Can you work these out from the model? Positions are in its coordinate system, mm. A direction names the side the tool comes from. Coordinates: 2 decimals unless noted, no trailing zeros. Loops run counter-clockwise (first coordinate to the right, second up) from the corner with the lowest first, then second, coordinate; pieces in that order, holes last. Notation, with made-up numbers: (-19.5, 7) - (-4.5, 7) arc R22 cw to (-4.5, 36) - close; hole circle Ø9 at (32, 66.25). An arc over 180 degrees is marked (long way). Put each result on its own line as item: value. Start each with the question number.
from build123d import *

# Parameters (mm, degrees)
SKETCH_1_W                  = 230
SKETCH_1_H                  = 150
EXTRUDE_1_DEPTH             = 20
SKETCH_2_W                  = 110
SKETCH_2_H                  = 20
EXTRUDE_2_DEPTH             = 135
FILLET_1_R                  = 55
SKETCH_4_R                  = 27.5
CUT_EXTRUDE_1_DEPTH         = 233.701525564
SKETCH_5_R                  = 11
CUT_EXTRUDE_2_DEPTH         = 193.54869514
PATTERN_LINEAR_1_COUNT      = 2
PATTERN_LINEAR_1_PITCH      = 180
PATTERN_LINEAR_1_COUNT_DIR2 = 2
PATTERN_LINEAR_1_PITCH_DIR2 = 100


with BuildPart() as part:
    # 草图1 → 凸台-拉伸1 (new body)
    with BuildSketch(Plane(origin=(0, 0, 0), x_dir=(1, 0, 0), z_dir=(0, 1, 0))):
        Rectangle(SKETCH_1_W, SKETCH_1_H)
    extrude(amount=EXTRUDE_1_DEPTH)

    # 草图2 → 凸台-拉伸2 (add)
    with BuildSketch(Plane(origin=(0, 20, 0), x_dir=(1, 0, 0), z_dir=(0, 1, 0))):
        with Locations((0, 45)):
            Rectangle(SKETCH_2_W, SKETCH_2_H)
    extrude_2 = extrude(amount=EXTRUDE_2_DEPTH)

    # 镜向1: 凸台-拉伸2 across plane
    add(extrude_2.mirror(Plane.XY))

    # 圆角1
    fillet_1_edges = [part.edges().sort_by_distance(p)[0] for p in [
        (-55, 155, -45),
        (55, 155, -45),
        (-55, 155, 45),
        (55, 155, 45),
    ]]
    fillet(fillet_1_edges, radius=FILLET_1_R - 0.0001)  # a hair under: the kernel refuses the full size

    # 草图4 → 切除-拉伸1 (cut, through all)
    with BuildSketch(Plane.XY.offset(55)):
        with Locations((0, 100)):
            Circle(SKETCH_4_R)
    extrude(amount=-CUT_EXTRUDE_1_DEPTH, mode=Mode.SUBTRACT)

    # 草图5 → 切除-拉伸2 (cut, through all)
    with BuildSketch(Plane(origin=(0, 20, 0), x_dir=(1, 0, 0), z_dir=(0, 1, 0))):
        with Locations(Location((-90, 50, 0), (0, 0, 270))):
            Circle(SKETCH_5_R)
    cut_extrude_2 = extrude(amount=-CUT_EXTRUDE_2_DEPTH, mode=Mode.SUBTRACT)

    # 阵列(线性)1: Cut-Extrude 2 2 × 2
    with Locations(*[(i * PATTERN_LINEAR_1_PITCH, 0, j * PATTERN_LINEAR_1_PITCH_DIR2) for i in range(PATTERN_LINEAR_1_COUNT) for j in range(PATTERN_LINEAR_1_COUNT_DIR2) if (i, j) != (0, 0)]):
        add(cut_extrude_2, mode=Mode.SUBTRACT)


solid = part.part
Q1. Please list where these lines run through material, in increasing order: line 1 along Z through (x, y) = (-8.5, 26); line 2 along Y through (x, z) = (0, 48.25); line 3 along Y through (x, z) = (-60.5, -31.5). Write a range as [from, to].
Q2. I want a section at B-B on z = -50. Count the separate pieces of the cut face and the enclosed holes in it, and give its area (3 significant figures).
Q3. Will these pins go through, and if not, where does the flat tip stop? pin 1 (22 mm diameter, centred on y = 67, z = 50, fed in from +X); pin 2 (1 mm diameter, centred on x = 13, y = 30, fed in from -Z); pin 3 (10 mm diameter, centred on y = 61.5, z = 45, fed in from -X).
Q4. I want a section at D-D on y = 136. List the corners of the cut face in (x, z) for me.
Q5. We'd pull the mould along Z, two halves only. Please class faces 1 (the flat face through (-115, 10, 1)), 2 (the cylindrical face through (-79.094, 10.14, -51.432)), 3 (the flat face through (-2, 10, 75)): released by +Z, released by -Z, zero draft, split by the parting line, or undercut.
Q6. I want a section at A-A on x = 90. List the corners of the cut face in (y, z) for me.
Q7. I want a section at C-C on y = 92. List the corners of the cut face in (x, z) for me.
Q8. On a 3-axis mill with a long thin cutter (end or side, diameter ignored), from which of +Z, -Z, +X, -X, +Y, -Y can I reach the whole of each face in a straight line? I mean faces 4 (the flat face through (-55, 59, 45)), 5 (the flat face through (-1, 72, -55)), 6 (the flat face through (-1, 72, -35)). Say none if no direction works.
Calculated:
1. line 1: [-55, -35], [35, 55]
1. line 2: [0, 72.5], [127.5, 155]
1. line 3: [0, 20]
2. separate pieces: 3
2. enclosed holes: 1
2. area: 14,900 mm2
3. pin 1: x = 55
3. pin 2: z = -55
3. pin 3: x = -55
4. outline: (-41.58, -55) - (41.58, -55) - (41.58, -35) - (-41.58, -35) - close; (-41.58, 35) - (41.58, 35) - (41.58, 55) - (-41.58, 55) - close
5. face 1: zero draft
5. face 2: undercut
5. face 3: released by +Z
6. outline: (0, -75) - (20, -75) - (20, -61) - (0, -61) - close; (0, -39) - (20, -39) - (20, 39) - (0, 39) - close; (0, 61) - (20, 61) - (20, 75) - (0, 75) - close
7. outline: (-55, -55) - (-26.31, -55) - (-26.31, -35) - (-55, -35) - close; (-55, 35) - (-26.31, 35) - (-26.31, 55) - (-55, 55) - close; (26.31, -55) - (55, -55) - (55, -35) - (26.31, -35) - close; (26.31, 35) - (55, 35) - (55, 55) - (26.31, 55) - close
8. face 4: +Z, -Z, -X, +Y
8. face 5: -Z, +X, -X, +Y
8. face 6: +X, -X, +Y
